from build123d import *

# Parameters (mm, degrees)
SKETCH1_W                      = 1430
SKETCH1_H                      = 60
BOSS_EXTRUDE1_DEPTH            = 35
SKETCH2_W                      = 356
SKETCH2_H                      = 60
CUT_EXTRUDE1_DEPTH             = 35
M5X0_8_TAPPED_HOLE2_D          = 4.2
LPATTERN1_COUNT                = 13
LPATTERN1_PITCH                = 40
MIRROR1_COPY_1_D               = 4.2
MIRROR1_COPY_2_D               = 4.2
MIRROR1_COPY_3_D               = 4.2
MIRROR1_COPY_4_D               = 4.2
MIRROR1_COPY_5_D               = 4.2
MIRROR1_COPY_6_D               = 4.2
MIRROR1_COPY_7_D               = 4.2
MIRROR1_COPY_8_D               = 4.2
MIRROR1_COPY_9_D               = 4.2
MIRROR1_COPY_10_D              = 4.2
MIRROR1_COPY_11_D              = 4.2
MIRROR1_COPY_12_D              = 4.2
M4X0_7_TAPPED_HOLE1_AT_2_COUNT = 2
M4X0_7_TAPPED_HOLE1_AT_2_PITCH = 12
M4X0_7_TAPPED_HOLE1_AT_3_COUNT = 2
M4X0_7_TAPPED_HOLE1_AT_3_PITCH = 55
M4X0_7_TAPPED_HOLE1_AT_4_COUNT = 2
M4X0_7_TAPPED_HOLE1_AT_4_PITCH = 56.29387178
M4X0_7_TAPPED_HOLE1_AT_5_COUNT = 2
M4X0_7_TAPPED_HOLE1_AT_5_PITCH = 115
M4X0_7_TAPPED_HOLE1_AT_6_COUNT = 2
M4X0_7_TAPPED_HOLE1_AT_6_PITCH = 115.62439189
FILLET1_R                      = 10


with BuildPart() as part:
    # Sketch1 → Boss-Extrude1 (new body, symmetric)
    with BuildSketch(Plane(origin=(0, 0, 0), x_dir=(1, 0, 0), z_dir=(0, 1, 0))):
        Rectangle(SKETCH1_W, SKETCH1_H)
    extrude(amount=BOSS_EXTRUDE1_DEPTH, both=True)

    # Sketch2 → Cut-Extrude1 (cut)
    with BuildSketch(Plane(origin=(0, 35, 0), x_dir=(1, 0, 0), z_dir=(0, 1, 0))):
        Rectangle(SKETCH2_W, SKETCH2_H)
    extrude(amount=-CUT_EXTRUDE1_DEPTH, mode=Mode.SUBTRACT)

    # M5x0.8 Tapped Hole2 (through all)
    with Locations(Plane(origin=(0, 35, 0), x_dir=(1, 0, 0), z_dir=(0, 1, 0))):
        with Locations((205.9918251, 11.5), (205.9918251, -11.5)):
            m5x0_8_tapped_hole2 = Hole(M5X0_8_TAPPED_HOLE2_D / 2)

    # LPattern1: M5x0.8 Tapped Hole2 ×13
    with Locations(*[(i * LPATTERN1_PITCH, 0, 0) for i in range(1, LPATTERN1_COUNT)]):
        add(m5x0_8_tapped_hole2, mode=Mode.SUBTRACT)

    # Mirror1: M5x0.8 Tapped Hole2 across plane
    add(m5x0_8_tapped_hole2.mirror(Plane(origin=(0, 0, 0), x_dir=(0, 0, 1), z_dir=(1, 0, 0))), mode=Mode.SUBTRACT)

    # Mirror1 copy 1 (through all)
    with Locations(Plane(origin=(-40, 35, 0), x_dir=(-1, 0, 0), z_dir=(0, 1, 0))):
        with Locations((205.9918251, -11.5), (205.9918251, 11.5)):
            Hole(MIRROR1_COPY_1_D / 2)

    # Mirror1 copy 2 (through all)
    with Locations(Plane(origin=(-80, 35, 0), x_dir=(-1, 0, 0), z_dir=(0, 1, 0))):
        with Locations((205.9918251, -11.5), (205.9918251, 11.5)):
            Hole(MIRROR1_COPY_2_D / 2)

    # Mirror1 copy 3 (through all)
    with Locations(Plane(origin=(-120, 35, 0), x_dir=(-1, 0, 0), z_dir=(0, 1, 0))):
        with Locations((205.9918251, -11.5), (205.9918251, 11.5)):
            Hole(MIRROR1_COPY_3_D / 2)

    # Mirror1 copy 4 (through all)
    with Locations(Plane(origin=(-160, 35, 0), x_dir=(-1, 0, 0), z_dir=(0, 1, 0))):
        with Locations((205.9918251, -11.5), (205.9918251, 11.5)):
            Hole(MIRROR1_COPY_4_D / 2)

    # Mirror1 copy 5 (through all)
    with Locations(Plane(origin=(-200, 35, 0), x_dir=(-1, 0, 0), z_dir=(0, 1, 0))):
        with Locations((205.9918251, -11.5), (205.9918251, 11.5)):
            Hole(MIRROR1_COPY_5_D / 2)

    # Mirror1 copy 6 (through all)
    with Locations(Plane(origin=(-240, 35, 0), x_dir=(-1, 0, 0), z_dir=(0, 1, 0))):
        with Locations((205.9918251, -11.5), (205.9918251, 11.5)):
            Hole(MIRROR1_COPY_6_D / 2)

    # Mirror1 copy 7 (through all)
    with Locations(Plane(origin=(-280, 35, 0), x_dir=(-1, 0, 0), z_dir=(0, 1, 0))):
        with Locations((205.9918251, -11.5), (205.9918251, 11.5)):
            Hole(MIRROR1_COPY_7_D / 2)

    # Mirror1 copy 8 (through all)
    with Locations(Plane(origin=(-320, 35, 0), x_dir=(-1, 0, 0), z_dir=(0, 1, 0))):
        with Locations((205.9918251, -11.5), (205.9918251, 11.5)):
            Hole(MIRROR1_COPY_8_D / 2)

    # Mirror1 copy 9 (through all)
    with Locations(Plane(origin=(-360, 35, 0), x_dir=(-1, 0, 0), z_dir=(0, 1, 0))):
        with Locations((205.9918251, -11.5), (205.9918251, 11.5)):
            Hole(MIRROR1_COPY_9_D / 2)

    # Mirror1 copy 10 (through all)
    with Locations(Plane(origin=(-400, 35, 0), x_dir=(-1, 0, 0), z_dir=(0, 1, 0))):
        with Locations((205.9918251, -11.5), (205.9918251, 11.5)):
            Hole(MIRROR1_COPY_10_D / 2)

    # Mirror1 copy 11 (through all)
    with Locations(Plane(origin=(-440, 35, 0), x_dir=(-1, 0, 0), z_dir=(0, 1, 0))):
        with Locations((205.9918251, -11.5), (205.9918251, 11.5)):
            Hole(MIRROR1_COPY_11_D / 2)

    # Mirror1 copy 12 (through all)
    with Locations(Plane(origin=(-480, 35, 0), x_dir=(-1, 0, 0), z_dir=(0, 1, 0))):
        with Locations((205.9918251, -11.5), (205.9918251, 11.5)):
            Hole(MIRROR1_COPY_12_D / 2)

    # Sketch10 → M4x0.7 Tapped Hole1 (revolve, cut)
    with BuildSketch(Plane(origin=(142.5, -17.5, 30), x_dir=(0, -1, 0), z_dir=(1, 0, 0))):
        Polygon((0, 0), (0, 15.991420021), (1.65, 15), (1.65, 0), align=None)
    m4x0_7_tapped_hole1 = revolve(axis=Axis((142.5, -17.5, 36.35), (0, 0, -1)), mode=Mode.SUBTRACT)

    # M4x0.7 Tapped Hole1 at 2: M4x0.7 Tapped Hole1 ×2
    with Locations(*[(0, -i * M4X0_7_TAPPED_HOLE1_AT_2_PITCH, 0) for i in range(1, M4X0_7_TAPPED_HOLE1_AT_2_COUNT)]):
        add(m4x0_7_tapped_hole1, mode=Mode.SUBTRACT)

    # M4x0.7 Tapped Hole1 at 3: M4x0.7 Tapped Hole1 ×2
    with Locations(*[(-i * M4X0_7_TAPPED_HOLE1_AT_3_PITCH, 0, 0) for i in range(1, M4X0_7_TAPPED_HOLE1_AT_3_COUNT)]):
        add(m4x0_7_tapped_hole1, mode=Mode.SUBTRACT)

    # M4x0.7 Tapped Hole1 at 4: M4x0.7 Tapped Hole1 ×2
    with Locations(*[Vector(-0.977015761, -0.213167075, 0) * (i * M4X0_7_TAPPED_HOLE1_AT_4_PITCH) for i in range(1, M4X0_7_TAPPED_HOLE1_AT_4_COUNT)]):
        add(m4x0_7_tapped_hole1, mode=Mode.SUBTRACT)

    # M4x0.7 Tapped Hole1 at 5: M4x0.7 Tapped Hole1 ×2
    with Locations(*[(-i * M4X0_7_TAPPED_HOLE1_AT_5_PITCH, 0, 0) for i in range(1, M4X0_7_TAPPED_HOLE1_AT_5_COUNT)]):
        add(m4x0_7_tapped_hole1, mode=Mode.SUBTRACT)

    # M4x0.7 Tapped Hole1 at 6: M4x0.7 Tapped Hole1 ×2
    with Locations(*[Vector(-0.994599826, -0.10378433, 0) * (i * M4X0_7_TAPPED_HOLE1_AT_6_PITCH) for i in range(1, M4X0_7_TAPPED_HOLE1_AT_6_COUNT)]):
        add(m4x0_7_tapped_hole1, mode=Mode.SUBTRACT)

    # Mirror2: M4x0.7 Tapped Hole1 across plane
    add(m4x0_7_tapped_hole1.mirror(Plane(origin=(0, 0, 0), x_dir=(0, 0, 1), z_dir=(1, 0, 0))), mode=Mode.SUBTRACT)

    # Mirror2 copy 1 sketch → Mirror2 copy 1 (revolve, cut)
    with BuildSketch(Plane(origin=(-142.5, -29.5, 30), x_dir=(0, -1, 0), z_dir=(-1, 0, 0))):
        Polygon((0, 0), (0, -15.991420021), (1.65, -15), (1.65, 0), align=None)
    revolve(axis=Axis((-142.5, -29.5, 36.35), (0, 0, 1)), mode=Mode.SUBTRACT)

    # Mirror2 copy 2 sketch → Mirror2 copy 2 (revolve, cut)
    with BuildSketch(Plane(origin=(-87.5, -17.5, 30), x_dir=(0, -1, 0), z_dir=(-1, 0, 0))):
        Polygon((0, 0), (0, -15.991420021), (1.65, -15), (1.65, 0), align=None)
    revolve(axis=Axis((-87.5, -17.5, 36.35), (0, 0, 1)), mode=Mode.SUBTRACT)

    # Mirror2 copy 3 sketch → Mirror2 copy 3 (revolve, cut)
    with BuildSketch(Plane(origin=(-87.5, -29.5, 30), x_dir=(0, -1, 0), z_dir=(-1, 0, 0))):
        Polygon((0, 0), (0, -15.991420021), (1.65, -15), (1.65, 0), align=None)
    revolve(axis=Axis((-87.5, -29.5, 36.35), (0, 0, 1)), mode=Mode.SUBTRACT)

    # Mirror2 copy 4 sketch → Mirror2 copy 4 (revolve, cut)
    with BuildSketch(Plane(origin=(-27.5, -17.5, 30), x_dir=(0, -1, 0), z_dir=(-1, 0, 0))):
        Polygon((0, 0), (0, -15.991420021), (1.65, -15), (1.65, 0), align=None)
    revolve(axis=Axis((-27.5, -17.5, 36.35), (0, 0, 1)), mode=Mode.SUBTRACT)

    # Mirror2 copy 5 sketch → Mirror2 copy 5 (revolve, cut)
    with BuildSketch(Plane(origin=(-27.5, -29.5, 30), x_dir=(0, -1, 0), z_dir=(-1, 0, 0))):
        Polygon((0, 0), (0, -15.991420021), (1.65, -15), (1.65, 0), align=None)
    revolve(axis=Axis((-27.5, -29.5, 36.35), (0, 0, 1)), mode=Mode.SUBTRACT)

    # Mirror3: M4x0.7 Tapped Hole1 across plane
    add(m4x0_7_tapped_hole1.mirror(Plane.XY), mode=Mode.SUBTRACT)

    # Mirror3 copy 1 sketch → Mirror3 copy 1 (revolve, cut)
    with BuildSketch(Plane(origin=(-142.5, -17.5, -30), x_dir=(0, -1, 0), z_dir=(-1, 0, 0))):
        Polygon((0, 0), (0, 15.991420021), (1.65, 15), (1.65, 0), align=None)
    revolve(axis=Axis((-142.5, -17.5, -36.35), (0, 0, 1)), mode=Mode.SUBTRACT)

    # Mirror3 copy 2 sketch → Mirror3 copy 2 (revolve, cut)
    with BuildSketch(Plane(origin=(-142.5, -29.5, -30), x_dir=(0, -1, 0), z_dir=(-1, 0, 0))):
        Polygon((0, 0), (0, 15.991420021), (1.65, 15), (1.65, 0), align=None)
    revolve(axis=Axis((-142.5, -29.5, -36.35), (0, 0, 1)), mode=Mode.SUBTRACT)

    # Mirror3 copy 3 sketch → Mirror3 copy 3 (revolve, cut)
    with BuildSketch(Plane(origin=(-87.5, -17.5, -30), x_dir=(0, -1, 0), z_dir=(-1, 0, 0))):
        Polygon((0, 0), (0, 15.991420021), (1.65, 15), (1.65, 0), align=None)
    revolve(axis=Axis((-87.5, -17.5, -36.35), (0, 0, 1)), mode=Mode.SUBTRACT)

    # Mirror3 copy 4 sketch → Mirror3 copy 4 (revolve, cut)
    with BuildSketch(Plane(origin=(-87.5, -29.5, -30), x_dir=(0, -1, 0), z_dir=(-1, 0, 0))):
        Polygon((0, 0), (0, 15.991420021), (1.65, 15), (1.65, 0), align=None)
    revolve(axis=Axis((-87.5, -29.5, -36.35), (0, 0, 1)), mode=Mode.SUBTRACT)

    # Mirror3 copy 5 sketch → Mirror3 copy 5 (revolve, cut)
    with BuildSketch(Plane(origin=(-27.5, -17.5, -30), x_dir=(0, -1, 0), z_dir=(-1, 0, 0))):
        Polygon((0, 0), (0, 15.991420021), (1.65, 15), (1.65, 0), align=None)
    revolve(axis=Axis((-27.5, -17.5, -36.35), (0, 0, 1)), mode=Mode.SUBTRACT)

    # Mirror3 copy 6 sketch → Mirror3 copy 6 (revolve, cut)
    with BuildSketch(Plane(origin=(-27.5, -29.5, -30), x_dir=(0, -1, 0), z_dir=(-1, 0, 0))):
        Polygon((0, 0), (0, 15.991420021), (1.65, 15), (1.65, 0), align=None)
    revolve(axis=Axis((-27.5, -29.5, -36.35), (0, 0, 1)), mode=Mode.SUBTRACT)

    # Mirror3 copy 7 sketch → Mirror3 copy 7 (revolve, cut)
    with BuildSketch(Plane(origin=(142.5, -29.5, -30), x_dir=(0, -1, 0), z_dir=(1, 0, 0))):
        Polygon((0, 0), (0, -15.991420021), (1.65, -15), (1.65, 0), align=None)
    revolve(axis=Axis((142.5, -29.5, -36.35), (0, 0, -1)), mode=Mode.SUBTRACT)

    # Mirror3 copy 8 sketch → Mirror3 copy 8 (revolve, cut)
    with BuildSketch(Plane(origin=(87.5, -17.5, -30), x_dir=(0, -1, 0), z_dir=(1, 0, 0))):
        Polygon((0, 0), (0, -15.991420021), (1.65, -15), (1.65, 0), align=None)
    revolve(axis=Axis((87.5, -17.5, -36.35), (0, 0, -1)), mode=Mode.SUBTRACT)

    # Mirror3 copy 9 sketch → Mirror3 copy 9 (revolve, cut)
    with BuildSketch(Plane(origin=(87.5, -29.5, -30), x_dir=(0, -1, 0), z_dir=(1, 0, 0))):
        Polygon((0, 0), (0, -15.991420021), (1.65, -15), (1.65, 0), align=None)
    revolve(axis=Axis((87.5, -29.5, -36.35), (0, 0, -1)), mode=Mode.SUBTRACT)

    # Mirror3 copy 10 sketch → Mirror3 copy 10 (revolve, cut)
    with BuildSketch(Plane(origin=(27.5, -17.5, -30), x_dir=(0, -1, 0), z_dir=(1, 0, 0))):
        Polygon((0, 0), (0, -15.991420021), (1.65, -15), (1.65, 0), align=None)
    revolve(axis=Axis((27.5, -17.5, -36.35), (0, 0, -1)), mode=Mode.SUBTRACT)

    # Mirror3 copy 11 sketch → Mirror3 copy 11 (revolve, cut)
    with BuildSketch(Plane(origin=(27.5, -29.5, -30), x_dir=(0, -1, 0), z_dir=(1, 0, 0))):
        Polygon((0, 0), (0, -15.991420021), (1.65, -15), (1.65, 0), align=None)
    revolve(axis=Axis((27.5, -29.5, -36.35), (0, 0, -1)), mode=Mode.SUBTRACT)

    # Fillet1
    fillet1_edges = [part.edges().sort_by_distance(p)[0] for p in [
        (715, 35, 0),
        (-715, 35, 0),
    ]]
    fillet(fillet1_edges, radius=FILLET1_R)


solid = part.part
Build history of the part. All positions in model axes, mm. A direction names the side the tool comes from. Round coordinates to 2 decimals unless told otherwise and drop trailing zeros. Answer in a Markdown table with one row per item.
1. Mould opens along X. For faces 1 (the face through (-715, -5, 0)), 2 (the face through (715, -5, 0)), 3 (the face through (-178, 18, 0)), 4 (the face through (-10, -7, -30)) say: +X half, -X half, draft (parallel to the pull), parting line (faces both ways), or undercut.
Geometry check:
| item | result |
|---|---|
| face 1 | -X half |
| face 2 | +X half |
| face 3 | undercut |
| face 4 | draft |
2. Probe L1, parallel to Z at x = 525, y = -11; L2, parallel to Z at x = 327, y = -6; L3, parallel to X at y = 13, z = 18. List the from-to ranges inside material, lowest first. Write a range as [from, to].
Geometry check:
| item | result |
|---|---|
| L1 | [-30, -13.35], [-9.65, 9.65], [13.35, 30] |
| L2 | [-30, -13.34], [-9.66, 9.66], [13.34, 30] |
| L3 | [-715, -178], [178, 715] |
3. Flat gauge pin, fed straight in: P1, Ø10, axis at x = -95, z = 21.5, coming from the +Y side. Where does the tip first touch, or does it go through?
Geometry check:
| item | result |
|---|---|
| P1 | y = 0 |
4. Which spindle directions (+Z, -Z, +X, -X, +Y, -Y) get a long thin tool onto all of the face, cutting with end or side? Do faces 5 (the face through (-2, 0, 0)), 6 (the face through (-10, -35, 0)). Say none if no direction does.
Geometry check:
| item | result |
|---|---|
| face 5 | +Z, -Z, +Y |
| face 6 | +Z, -Z, +X, -X, -Y |
